from build123d import *

# Parameters (mm, degrees)
BOSS_EXTRUDE1_DEPTH = 3


with BuildPart() as part:
    # Sketch1 → Boss-Extrude1 (new body)
    with BuildSketch(Plane(origin=(0, 0, 0), x_dir=(0, 1, 0), z_dir=(0, 0, 1))):
        with BuildLine():
            Line((-26.9, 13.95), (-24.9, 13.95))
            Line((-24.9, 13.95), (-24.9, 15.95))
            Line((-24.9, 15.95), (-26.9, 15.95))
            ThreePointArc((-26.9, 15.95), (-31.213351365, 14.163351365), (-33, 9.85))
            Line((-33, 9.85), (-33, -9.85))
            ThreePointArc((-33, -9.85), (-31.213351365, -14.163351365), (-26.9, -15.95))
            Line((-26.9, -15.95), (26.9, -15.95))
            ThreePointArc((26.9, -15.95), (31.213351365, -14.163351365), (33, -9.85))
            Line((33, -9.85), (33, 9.85))
            ThreePointArc((33, 9.85), (31.213351365, 14.163351365), (26.9, 15.95))
            Line((26.9, 15.95), (24.9, 15.95))
            Line((24.9, 15.95), (24.9, 13.95))
            Line((24.9, 13.95), (26.9, 13.95))
            ThreePointArc((26.9, 13.95), (29.799137803, 12.749137803), (31, 9.85))
            Line((31, 9.85), (31, -9.85))
            ThreePointArc((31, -9.85), (29.799137803, -12.749137803), (26.9, -13.95))
            Line((26.9, -13.95), (-26.9, -13.95))
            ThreePointArc((-26.9, -13.95), (-29.799137803, -12.749137803), (-31, -9.85))
            Line((-31, -9.85), (-31, 9.85))
            ThreePointArc((-31, 9.85), (-29.799137803, 12.749137803), (-26.9, 13.95))
        make_face()
    extrude(amount=BOSS_EXTRUDE1_DEPTH)


solid = part.part
Design review of the part built by this model. Coordinates are the model's own, in mm. A direction names the side the tool comes from. Give positions to 0.01 mm unless a question says otherwise; leave off trailing zeros. Order: outer loops, then holes, each group sorted by start corner. A loop starts at its lowest first (then second) coordinate and runs counter-clockwise, first axis right, second up. Notation, with made-up numbers: (78, 3) - (125, 3) arc R32 ccw to (125, 30) - close; hole circle Ø2 at (79.5, 15). An arc over 180 degrees is marked (long way). Use CSV: the item, a comma, the result in double quotes. Start each with the question number.
Q1. Take a section at D-D (x = -11.5). State the section outline as (y, z) points, and give its area (3 significant figures).
Q2. Draft analysis for pull direction Y (two halves, no side actions). For faces 1 (the face through (0, -33, 1)), 2 (the face through (14.1, -0.2, 3)), 3 (the face through (12.72, 29.83, 1.48)), state which applies: pulls with the +Y half, pulls with the -Y half, needs draft (parallel to the pull), parting line crosses it, or undercut.
Q3. Take a section at A-A (x = -6.5). State the section outline as (y, z) points.
Q4. Take a section at B-B (z = 1.4). State the section outline as (x, y) points, and give its area (3 significant figures).
Q5. Take a section at C-C (y = -22). State the section outline as (x, z) points, and give its area (3 significant figures).
Q6. For line 1 (Y direction, x = -2, z = 2.3); line 2 (X direction, y = -23.5, z = 2.45); line 3 (Y direction, x = -12.5, z = 2.6), list the stretches that pass through material, from the lowest coordinate up.
Q7. For P1, Ø1, axis at x = -15, z = 1.5, coming from the +Y side; P2, Ø1.6, axis at x = -15, z = 2, coming from the -Y side; P3, Ø1.5, axis at y = -12.5, z = 2, coming from the -X side, all flat-tipped, find the tip position at first contact; note any pin that passes through.
Q8. Machinability: for faces 4 (the face through (-15, 24.9, 1)), 5 (the face through (-12.72, -29.83, 1.48)), 6 (the face through (-14.116, 31.261, 1.479)), which of the approach directions +Z, -Z, +X, -X, +Y, -Y give a long, thin tool a straight path to every point of the face, cutting with its end or side? Answer none if there is none.
Calculated:
1,outline,"(-32.77, 0) - (-30.65, 0) - (-30.65, 3) - (-32.77, 3) - close; (30.65, 0) - (32.77, 0) - (32.77, 3) - (30.65, 3) - close"
1,area,"12.7 mm²"
2,face 1,"pulls with the -Y half"
2,face 2,"needs draft"
2,face 3,"undercut"
3,outline,"(-33, 0) - (-31, 0) - (-31, 3) - (-33, 3) - close; (31, 0) - (33, 0) - (33, 3) - (31, 3) - close"
4,outline,"(-15.95, -26.9) arc R6.1 ccw to (-9.85, -33) - (9.85, -33) arc R6.1 ccw to (15.95, -26.9) - (15.95, 26.9) arc R6.1 ccw to (9.85, 33) - (-9.85, 33) arc R6.1 ccw to (-15.95, 26.9) - (-15.95, 24.9) - (-13.95, 24.9) - (-13.95, 26.9) arc R4.1 cw to (-9.85, 31) - (9.85, 31) arc R4.1 cw to (13.95, 26.9) - (13.95, -26.9) arc R4.1 cw to (9.85, -31) - (-9.85, -31) arc R4.1 cw to (-13.95, -26.9) - (-13.95, -24.9) - (-15.95, -24.9) - close"
4,area,"258 mm²"
5,outline,"(13.95, 0) - (15.95, 0) - (15.95, 3) - (13.95, 3) - close"
5,area,"6.00 mm²"
6,line 1,"y = -33 to -31, 31 to 33"
6,line 2,"x = 13.95 to 15.95"
6,line 3,"y = -32.39 to -30.03, 30.03 to 32.39"
7,P1,"stops at y = 30.85"
7,P2,"stops at y = -31.18"
7,P3,"stops at x = 13.95"
8,face 4,"+Z, -Z, -X"
8,face 5,"+Z, -Z"
8,face 6,"+Z, -Z, -X, +Y"
